Design review of the part built by this model. Coordinates are the model's own, in mm. Face numbers are marked on the shaded views. Give positions to 0.01 mm unless a question says otherwise; leave off trailing zeros. Write each loop counter-clockwise with the first axis right and the second up, starting at its lowest first coordinate (ties: lowest second). Pieces come first, ordered by that corner, then holes.
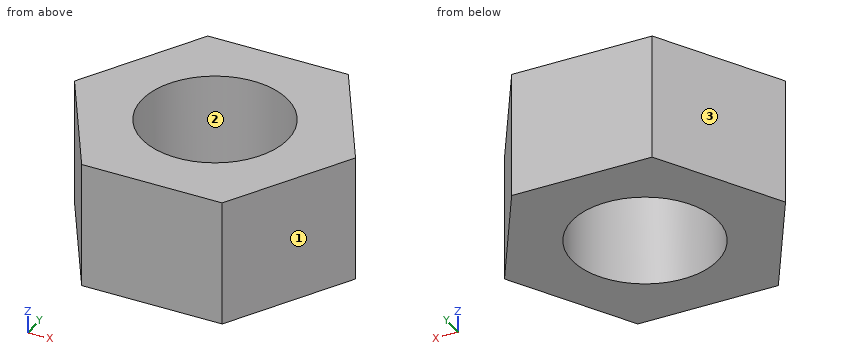
```python
from build123d import *

# Parameters (mm, degrees)
BOSS_EXTRUDE1_DEPTH = 2.6
SKETCH2_R           = 3
CUT_EXTRUDE1_DEPTH  = 6.2


with BuildPart() as part:
    # Sketch1 → Boss-Extrude1 (new body, symmetric)
    with BuildSketch(Plane.XY):
        Polygon((5.773502692, 0), (2.886751346, 5), (-2.886751346, 5), (-5.773502692, 0), (-2.886751346, -5), (2.886751346, -5), align=None)
    extrude(amount=BOSS_EXTRUDE1_DEPTH, both=True)

    # Sketch2 → Cut-Extrude1 (cut, through all)
    with BuildSketch(Plane.XY.offset(2.6)):
        Circle(SKETCH2_R)
    extrude(amount=-CUT_EXTRUDE1_DEPTH, mode=Mode.SUBTRACT)


solid = part.part
```
(1) Consider section B-B, the plane z = 1. Give the boundary of the cut face in (x, y).
Resolved:
outline: (-5.77, 0) - (-2.89, -5) - (2.89, -5) - (5.77, 0) - (2.89, 5) - (-2.89, 5) - close; hole circle Ø6 at (0, 0)
(2) Mouldability with a two-part tool opening along X and no side actions: class the marked faces 1, 2 and 3 as pulls with the +X half, pulls with the -X half, needs draft (parallel to the pull), parting line crosses it, or undercut.
Resolved:
face 1: pulls with the +X half
face 2: undercut
face 3: pulls with the -X half
(3) Consider section D-D, the plane y = 3.25. Give the boundary of the cut face in (x, z), then the cut area to 3 significant figures.
Resolved:
outline: (-3.9, -2.6) - (3.9, -2.6) - (3.9, 2.6) - (-3.9, 2.6) - close
area: 40.5 mm2
(4) Consider section A-A, the plane x = 0. Give the boundary of the cut face in (y, z).
Resolved:
outline: (-5, -2.6) - (-3, -2.6) - (-3, 2.6) - (-5, 2.6) - close; (3, -2.6) - (5, -2.6) - (5, 2.6) - (3, 2.6) - close
(5) Consider section C-C, the plane y = 0.75. Give the boundary of the cut face in (x, z).
Resolved:
outline: (-5.34, -2.6) - (-2.9, -2.6) - (-2.9, 2.6) - (-5.34, 2.6) - close; (2.9, -2.6) - (5.34, -2.6) - (5.34, 2.6) - (2.9, 2.6) - close
(6) To check wall thickness, follow L1, parallel to Y at x = 0, z = 0.3; L2, parallel to X at y = -1.5, z = -0.8; L3, parallel to X at y = 2, z = 0.9. State the ranges of each line that lie inside material, in increasing order.
Resolved:
L1: y = -5 to -3, 3 to 5
L2: x = -4.91 to -2.6, 2.6 to 4.91
L3: x = -4.62 to -2.24, 2.24 to 4.62
(7) Clearance check with flat-ended pins moving along their axes: P1, Ø3, axis at y = 3, z = -0.5, coming from the -X side; P2, Ø1.5, axis at y = -1.5, z = 0.5, coming from the +X side. State where each tip first meets the part, or that it passes through.
Resolved:
P1: stops at x = -4.91
P2: stops at x = 5.34
